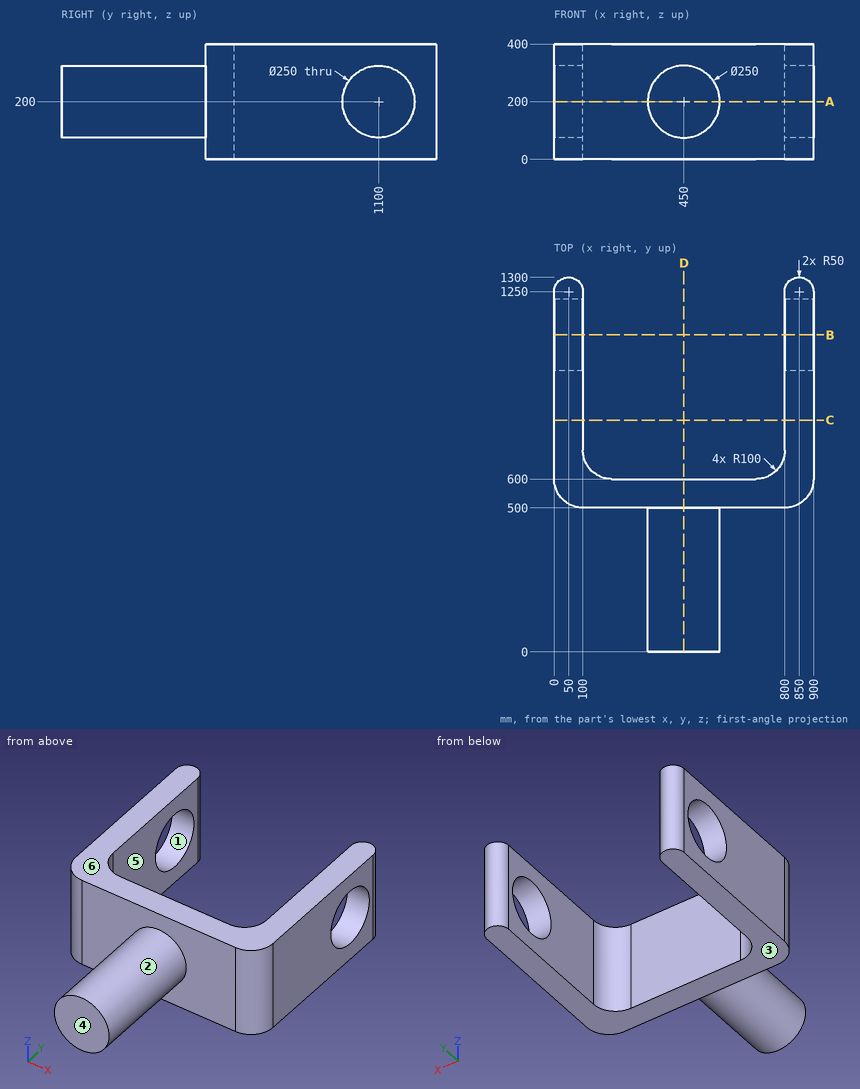
Source: three-view drawing plus pictorial views. Frame: mm from the lowest corner of the part. A direction names the side the tool comes from. Coordinates: 2 decimals unless noted, no trailing zeros. Loops run counter-clockwise (first coordinate to the right, second up) from the corner with the lowest first, then second, coordinate; pieces in that order, holes last. Notation, with made-up numbers: (-1, 43) -> (25, 43) arc R13 ccw to (25, 62) -> close; hole circle Ø4 at (-31.5, 57). An arc over 180 degrees is marked (long way). One line per item, written item: value.
(1) Ray query, line 1 along X through (y, z) = (850, 276.5); line 2 along Z through (x, y) = (71.5, 1100); line 3 along Y through (x, z) = (209, 105.5). Return the intervals inside material, ascending.
Answer below:
line 1: x = 0 to 100, 800 to 900
line 2: z = 0 to 75, 325 to 400
line 3: y = 500 to 600
(2) Cut plane A-A (z = 200). Output: boundary loops of the cut face in (x, y).
Answer below:
outline: (0, 600) arc R100 ccw to (100, 500) -> (325, 500) -> (325, 0) -> (575, 0) -> (575, 500) -> (800, 500) arc R100 ccw to (900, 600) -> (900, 975) -> (800, 975) -> (800, 700) arc R100 cw to (700, 600) -> (200, 600) arc R100 cw to (100, 700) -> (100, 975) -> (0, 975) -> close; (0, 1225) -> (100, 1225) -> (100, 1250) arc R50 ccw to (0, 1250) -> close; (800, 1225) -> (900, 1225) -> (900, 1250) arc R50 ccw to (800, 1250) -> close
(3) Cut plane D-D (x = 450). Output: boundary loops of the cut face in (y, z).
Answer below:
outline: (0, 75) -> (500, 75) -> (500, 0) -> (600, 0) -> (600, 400) -> (500, 400) -> (500, 325) -> (0, 325) -> close
(4) Cut plane B-B (y = 1100). Output: boundary loops of the cut face in (x, z), then the cut area to 3 significant figures.
Answer below:
outline: (0, 0) -> (100, 0) -> (100, 75) -> (0, 75) -> close; (0, 325) -> (100, 325) -> (100, 400) -> (0, 400) -> close; (800, 0) -> (900, 0) -> (900, 75) -> (800, 75) -> close; (800, 325) -> (900, 325) -> (900, 400) -> (800, 400) -> close
area: 30,000 mm2
(5) Pin query (flat end, axial travel): pin 1 Ø5 at (x, z) = (121.5, 333) entering from -Y. Return the tip coordinate at first contact, or that it passes through.
Answer below:
pin 1: stops at y = 500
(6) Set-up query: the marked faces 5 and 6. Return all of +Z, -Z, +X, -X, +Y, -Y with unobstructed straight access to the full face (end or side cutting, diameter ignored); none if empty.
Answer below:
face 5: +Z, -Z, +Y
face 6: +Z, +X, -X, +Y, -Y
(7) Cut plane C-C (y = 804). Output: boundary loops of the cut face in (x, z), then the cut area to 3 significant figures.
Answer below:
outline: (0, 0) -> (100, 0) -> (100, 400) -> (0, 400) -> close; (800, 0) -> (900, 0) -> (900, 400) -> (800, 400) -> close
area: 80,000 mm2
(8) Draft query along Z for the marked faces 1, 2, 3 and 4. Return one class per face: pulls with the +Z half, pulls with the -Z half, needs draft (parallel to the pull), parting line crosses it, or undercut.
Answer below:
face 1: undercut
face 2: parting line crosses it
face 3: pulls with the -Z half
face 4: needs draft
